Read the model definition and answer for the solid it produces. Units are mm, in the model's axes. Round coordinates to 2 decimals unless told otherwise and drop trailing zeros. Write each loop counter-clockwise with the first axis right and the second up, starting at its lowest first coordinate (ties: lowest second). Pieces come first, ordered by that corner, then holes. Notation, with made-up numbers: M 11,60.5 L 58,60.5 A33 cw 58,92.5 Z; hole C -31.75,58 d9. An arc over 180 degrees is marked long. Use one line per item in the form item = value. Start each with the question number.
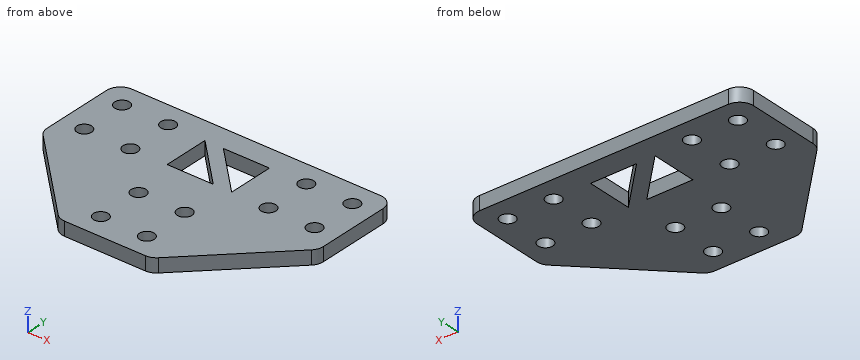
```python
from build123d import *

# Parameters (mm, degrees)
SKETCH_1_R      = 1.6
EXTRUDE_1_DEPTH = 3
FILLET_1_R      = 3


with BuildPart() as part:
    # 草图1 → 凸台-拉伸1 (new body)
    with BuildSketch(Plane.XY):
        Polygon((0, 0), (60, 0), (60, -20), (40, -40), (20, -40), (0, -20), align=None)
        with Locations((5, -5)):
            Circle(SKETCH_1_R, mode=Mode.SUBTRACT)
        with Locations(Location((15, -5, 0), (0, 0, 180))):
            Circle(SKETCH_1_R, mode=Mode.SUBTRACT)
        with Locations((15, -15)):
            Circle(SKETCH_1_R, mode=Mode.SUBTRACT)
        with Locations(Location((5, -15, 0), (0, 0, 180))):
            Circle(SKETCH_1_R, mode=Mode.SUBTRACT)
        with Locations((55, -15)):
            Circle(SKETCH_1_R, mode=Mode.SUBTRACT)
        with Locations(Location((45, -15, 0), (0, 0, 180))):
            Circle(SKETCH_1_R, mode=Mode.SUBTRACT)
        with Locations((45, -5)):
            Circle(SKETCH_1_R, mode=Mode.SUBTRACT)
        with Locations(Location((55, -5, 0), (0, 0, 180))):
            Circle(SKETCH_1_R, mode=Mode.SUBTRACT)
        with Locations((25, -35)):
            Circle(SKETCH_1_R, mode=Mode.SUBTRACT)
        with Locations(Location((35, -35, 0), (0, 0, 180))):
            Circle(SKETCH_1_R, mode=Mode.SUBTRACT)
        with Locations((35, -25)):
            Circle(SKETCH_1_R, mode=Mode.SUBTRACT)
        with Locations(Location((25, -25, 0), (0, 0, 180))):
            Circle(SKETCH_1_R, mode=Mode.SUBTRACT)
        Polygon((23, -5), (23, -15), (33, -15), align=None, mode=Mode.SUBTRACT)
        Polygon((27, -5), (37, -5), (37, -15), align=None, mode=Mode.SUBTRACT)
    extrude(amount=EXTRUDE_1_DEPTH)

    # 圆角1
    fillet_1_edges = [part.edges().sort_by_distance(p)[0] for p in [
        (0, 0, 1.5),
        (60, 0, 1.5),
        (60, -20, 1.5),
        (40, -40, 1.5),
        (20, -40, 1.5),
        (0, -20, 1.5),
    ]]
    fillet(fillet_1_edges, radius=FILLET_1_R)


solid = part.part
```
Q1. Find section C-C on z = 2.1. Count the separate pieces of the cut face and the enclosed holes in it, and give its area (3 significant figures).
Q2. Straight lines are drawn through the part: line 1 (X direction, y = -9.5, z = 1.5); line 2 (Y direction, x = 25, z = 2.2); line 3 (Y direction, x = 15, z = 1.3). For each, find the intervals that lie inside material, in ascending order. Write a range as [from, to].
Q3. Find section D-D on x = 55. Write down the section's boundary in (y, z), and give its area (3 significant figures).
Q4. Find section B-B on x = 35. Write down the section's boundary in (y, z).
Q5. Find section A-A on y = -25. Write down the section's boundary in (x, z).
Response:
q1.separate_pieces = 1
q1.enclosed_holes = 14
q1.area = 1,800 mm²
q2.line_1 = [0, 23], [27.5, 31.5], [37, 60]
q2.line_2 = [-40, -36.6], [-33.4, -26.6], [-23.4, -15], [-7, 0]
q2.line_3 = [-35, -16.6], [-13.4, -6.6], [-3.4, 0]
q3.outline = M -25,0 L -16.6,0 L -16.6,3 L -25,3 Z; M -13.4,0 L -6.6,0 L -6.6,3 L -13.4,3 Z; M -3.4,0 L 0,0 L 0,3 L -3.4,3 Z
q3.area = 55.8 mm²
q4.outline = M -40,0 L -36.6,0 L -36.6,3 L -40,3 Z; M -33.4,0 L -26.6,0 L -26.6,3 L -33.4,3 Z; M -23.4,0 L -13,0 L -13,3 L -23.4,3 Z; M -5,0 L 0,0 L 0,3 L -5,3 Z
q5.outline = M 5,0 L 23.4,0 L 23.4,3 L 5,3 Z; M 26.6,0 L 33.4,0 L 33.4,3 L 26.6,3 Z; M 36.6,0 L 55,0 L 55,3 L 36.6,3 Z
